from build123d import *

# Parameters (mm, degrees)
SKETCH1_R           = 71.85
SKETCH1_R_2         = 59.85
SKETCH1_R_3         = 1.65
BOSS_EXTRUDE1_DEPTH = 5


with BuildPart() as part:
    # Sketch1 → Boss-Extrude1 (new body)
    with BuildSketch(Plane.XY):
        Circle(SKETCH1_R)
        Circle(SKETCH1_R_2, mode=Mode.SUBTRACT)
        with Locations((66.5, 0)):
            Circle(SKETCH1_R_3, mode=Mode.SUBTRACT)
        with Locations((33.25, -57.590689352)):
            Circle(SKETCH1_R_3, mode=Mode.SUBTRACT)
        with Locations((-33.25, -57.590689352)):
            Circle(SKETCH1_R_3, mode=Mode.SUBTRACT)
        with Locations((-66.5, 0)):
            Circle(SKETCH1_R_3, mode=Mode.SUBTRACT)
        with Locations((-33.25, 57.590689352)):
            Circle(SKETCH1_R_3, mode=Mode.SUBTRACT)
        with Locations((33.25, 57.590689352)):
            Circle(SKETCH1_R_3, mode=Mode.SUBTRACT)
    extrude(amount=BOSS_EXTRUDE1_DEPTH)

    # Sketch2 → Cut-Revolve1 (revolve, cut)
    with BuildSketch(Plane(origin=(0, 0, 0), x_dir=(1, 0, 0), z_dir=(0, 1, 0)), mode=Mode.PRIVATE) as cut_revolve1_sk:
        Polygon((71.35, 0), (71.85, 0), (71.85, -5), align=None)
    revolve(cut_revolve1_sk.sketch.rotate(Axis((0, 0, 0), (0, 0, 1)), 180), axis=Axis((0, 0, 0), (0, 0, 1)), mode=Mode.SUBTRACT)


solid = part.part
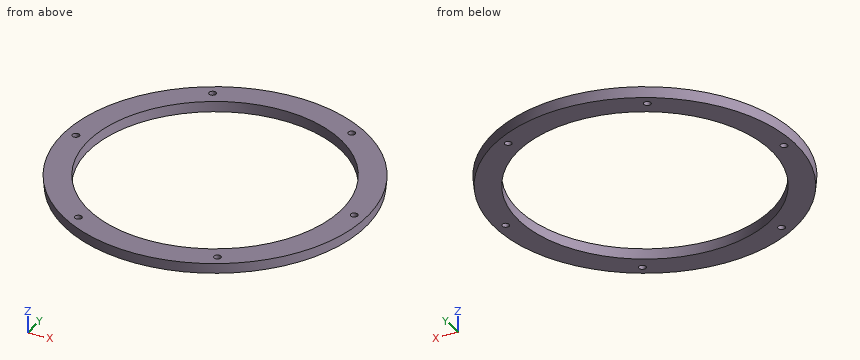
CAD build for the part. Positions are in the model's coordinates, mm. Give positions to 0.01 mm unless a question says otherwise; leave off trailing zeros. Write each loop counter-clockwise with the first axis right and the second up, starting at its lowest first coordinate (ties: lowest second). Pieces come first, ordered by that corner, then holes. Notation, with made-up numbers: (39, 33) - (97, 33) arc R32 cw to (97, 72) - close; hole circle Ø5 at (80.5, 0). An arc over 180 degrees is marked (long way). Put each result on its own line as item: value.
(1) Drop flat-ended pins along their axis: pin 1 Ø2 at (x, z) = (29, 3.5) entering from +Y; pin 2 Ø5.5 at (x, y) = (66.5, 0) entering from +Z; pin 3 Ø1 at (x, z) = (-25, 1.5) entering from -Y. Give the stop position or say it passes through.
Working result:
pin 1: y = 66.02
pin 2: z = 5
pin 3: y = -67.18
(2) Saw through at D-D (x = -33.25). Count the separate pieces of the cut face and the enclosed holes in it, then the cut area to 3 significant figures.
Working result:
separate pieces: 4
enclosed holes: 0
area: 103 mm^2
(3) Wall check: L1, parallel to Y at x = 33.25, z = 1.85; L2, parallel to X at y = -8, z = 0.7; L3, parallel to Y at x = -35, z = 3.6. Give the ranges that are in metal, low to high.
Working result:
L1: -63.34 to -59.24, -55.94 to -49.76, 49.76 to 55.94, 59.24 to 63.34
L2: -70.97 to -59.31, 59.31 to 70.97
L3: -62.59 to -48.55, 48.55 to 62.59
(4) Saw through at A-A (x = 0). List the corners of the cut face in (y, z), then the cut area to 4 significant figures.
Working result:
outline: (-71.85, 5) - (-71.35, 0) - (-59.85, 0) - (-59.85, 5) - close; (59.85, 0) - (71.35, 0) - (71.85, 5) - (59.85, 5) - close
area: 117.5 mm^2
(5) Saw through at C-C (z = 1.85). List the corners of the cut face in (x, y) (3 decimals).
Working result:
outline: circle Ø143.07 at (0, 0); hole circle Ø3.3 at (-66.5, 0); hole circle Ø119.7 at (0, 0); hole circle Ø3.3 at (-33.25, -57.591); hole circle Ø3.3 at (-33.25, 57.591); hole circle Ø3.3 at (33.25, -57.591); hole circle Ø3.3 at (33.25, 57.591); hole circle Ø3.3 at (66.5, 0)
(6) Saw through at B-B (y = 0). List the corners of the cut face in (x, z), then the cut area to 3 significant figures.
Working result:
outline: (-71.85, 5) - (-71.35, 0) - (-68.15, 0) - (-68.15, 5) - close; (-64.85, 0) - (-59.85, 0) - (-59.85, 5) - (-64.85, 5) - close; (59.85, 0) - (64.85, 0) - (64.85, 5) - (59.85, 5) - close; (68.15, 0) - (71.35, 0) - (71.85, 5) - (68.15, 5) - close
area: 84.5 mm^2
